The model under review builds one solid part; all positions refer to its coordinate system, in mm. A direction names the side the tool comes from. Coordinates: 2 decimals unless noted, no trailing zeros. Loops run counter-clockwise (first coordinate to the right, second up) from the corner with the lowest first, then second, coordinate; pieces in that order, holes last. Notation, with made-up numbers: M 23.5,53 L 72.5,53 A22 ccw 72.5,88 Z; hole C -28.75,39.25 d1. An arc over 180 degrees is marked long. Write item = value, one per line. Start each with the question number.
Q1. We need section B-B on x = 32. Give the boundary of the cut face in (y, z).
Q2. Mouldability with a two-part tool opening along Y and no side actions: class faces 1 (the face through (0.86, 61.1, 2.45)), 2 (the face through (49, 0, 3)), 3 (the face through (3.686, 57.334, 2.056)), 4 (the face through (53, 56, 6)) as released by +Y, released by -Y, zero draft, split by the parting line, or undercut.
Q3. Clearance check with flat-ended pins moving along their axes: pin 1 Ø1.7 at (x, y) = (96, 58.75) entering from +Z; pin 2 Ø4 at (x, y) = (70.5, 41.5) entering from -Z. State where each tip first meets the part, or that it passes through.
Q4. For faces 5 (the face through (49, 31, 0)), 6 (the face through (51, 6, 4)), 7 (the face through (100, 31, 3)), list the 3-axis set-ups (+Z, -Z, +X, -X, +Y, -Y) from which the entire face can be reached by the end or side of a thin tool; tool diameter is ignored.
Q5. We need section C-C on y = 50. Give the boundary of the cut face in (x, z).
Q6. We need section A-A on z = 5. Give the boundary of the cut face in (x, y), and give its area (3 significant figures).
Q7. Wall thickness on probe 1 along Y at (x, z) = (4, 1.5); probe 2 along Y at (x, z) = (86, 4.75); probe 3 along X at (y, z) = (17.5, 3): over which ranges is each line inside the solid? List them lowest first.
Autodesk Fusion 360 part; units mm, degrees
sketch "Sketch1" plane through (0, 0, 0) normal (0, 0, 1) x (1, 0, 0)
  line L0 (0, 0) -> (100, 0)
  line L1 (100, 0) -> (100, 62)
  line L2 (100, 62) -> (0, 62)
  line L3 (0, 62) -> (0, 0)
  line L4 (4, 55) -> (96, 55)
  line L5 (96, 55) -> (96, 6)
  line L6 (96, 6) -> (4, 6)
  line L7 (4, 6) -> (4, 55)
  dimension "d1" = 100
  dimension "d2" = 62
  dimension "d3" = 92
  dimension "d4" = 49
  dimension "d5" = 6
  dimension "d6" = 4
extrude "Extrude1" add sketch "Sketch1" along normal blind 2 contours L4 L5 L6 L7
extrude "Extrude2" add sketch "Sketch1" along normal blind 6
sketch "Sketch2" plane through (0, 0, 0) normal (0, 0, 1) x (1, 0, 0)
  line L0 (96, 52) -> (4, 52)
  line L1 (4, 52) -> (4, 10)
  line L2 (4, 10) -> (96, 10)
  line L3 (96, 10) -> (96, 52)
  line L4 (0, 0) -> (100, 0)
  line L5 (100, 0) -> (100, 62)
  dimension "d11" = 92
  dimension "d12" = 42
  dimension "d13" = 10
  dimension "d14" = 4
extrude "Extrude3" add sketch "Sketch1" against normal blind 2
ref_plane "WorkPlane1" through (0, 0, 15) normal (0, 0, 1) x (1, 0, 0)
sketch "Sketch3" plane through (0, 0, 15) normal (0, 0, 1) x (1, 0, 0)
  circle A0 centre (4, 3.25) radius 1.45
  circle A1 centre (96, 3.25) radius 1.45
  circle A2 centre (96, 58.75) radius 1.45
  circle A3 centre (4, 58.75) radius 1.45
  line L0 (0, 62) -> (0, 0)
  line L1 (0, 0) -> (100, 0)
  line L2 (100, 0) -> (100, 62)
  line L3 (100, 62) -> (0, 62)
  dimension "d18" = 2.9
  dimension "d19" = 2.9
  dimension "d20" = 2.9
  dimension "d21" = 2.9
  dimension "d22" = 4
  dimension "d23" = 3.25
  dimension "d24" = 4
  dimension "d25" = 3.25
  dimension "d26" = 4
  dimension "d27" = 3.25
  dimension "d28" = 4
  dimension "d29" = 3.25
extrude "Extrude4" cut sketch "Sketch3" against normal blind 25 contours A0 | A1 | A2 | A3
fillet "Fillet1" radius 3 4 edges at (100, 62, 2) (100, 0, 2) (0, 62, 2) (0, 0, 2)
fillet "Fillet2" radius 1 8 edges at (0.8787, 0.8787, -2) (0, 31, -2) (0.8787, 61.1213, -2) (50, 62, -2) (99.1213, 61.1213, -2) (100, 31, -2) (99.1213, 0.8787, -2) (50, 0, -2)
chamfer "Chamfer1" distance 1 angle 45 1 edges at (96, 30.5, -2)
chamfer "Chamfer2" distance 1 angle 45 1 edges at (4, 30.5, -2)
Returned:
q1.outline = M 0,-1 A1 ccw 1,-2 L 6,-2 L 6,0 L 55,0 L 55,-2 L 61,-2 A1 ccw 62,-1 L 62,6 L 55,6 L 55,2 L 6,2 L 6,6 L 0,6 Z
q2.face_1 = released by +Y
q2.face_2 = released by -Y
q2.face_3 = undercut
q2.face_4 = zero draft
q3.pin_1 = through
q3.pin_2 = 0
q4.face_5 = -Z
q4.face_6 = +Z
q4.face_7 = +Z, -Z, +X, +Y, -Y
q5.outline = M 0,-1 A1 ccw 1,-2 L 3,-2 L 4,-1 L 4,0 L 96,0 L 96,-1 L 97,-2 L 99,-2 A1 ccw 100,-1 L 100,6 L 96,6 L 96,2 L 4,2 L 4,6 L 0,6 Z
q6.outline = M 0,3 A3 ccw 3,0 L 97,0 A3 ccw 100,3 L 100,59 A3 ccw 97,62 L 3,62 A3 ccw 0,59 Z; hole C 4,3.25 d2.9; hole C 4,58.75 d2.9; hole M 4,6 L 96,6 L 96,55 L 4,55 Z; hole C 96,3.25 d2.9; hole C 96,58.75 d2.9
q6.area = 1,660 mm^2
q7.probe_1 = 0 to 1.8, 4.7 to 57.3, 60.2 to 62
q7.probe_2 = 0 to 6, 55 to 62
q7.probe_3 = 0 to 4, 96 to 100
